Work out the finished part from the listing and answer in its coordinate system (mm). Round coordinates to 2 decimals unless told otherwise and drop trailing zeros. Order: outer loops, then holes, each group sorted by start corner. A loop starts at its lowest first (then second) coordinate and runs counter-clockwise, first axis right, second up. Notation, with made-up numbers: (-14.5, 15.5) -> (-10.5, 15.5) arc R21 ccw to (-10.5, 23.5) -> close; hole circle Ø6 at (8, -37). An arc over 180 degrees is marked (long way). Use one line per item in the form item = value.
```python
from build123d import *

# Parameters (mm, degrees)
F1_DEPTH = 1206.5


with BuildPart() as f1:
    # F0 (on Front) → F1 (new body)
    with BuildSketch(Plane.XZ):
        with BuildLine():
            Line((0, 38.1), (0, 0))
            Line((0, 0), (38.1, 0))
            ThreePointArc((38.1, 0), (37.170064, 2.245064), (34.925, 3.175))
            Line((34.925, 3.175), (3.175, 3.175))
            Line((3.175, 3.175), (3.175, 34.925))
            ThreePointArc((3.175, 34.925), (2.245064, 37.170064), (0, 38.1))
        make_face()
    extrude(amount=-F1_DEPTH)


solid = f1.part
```
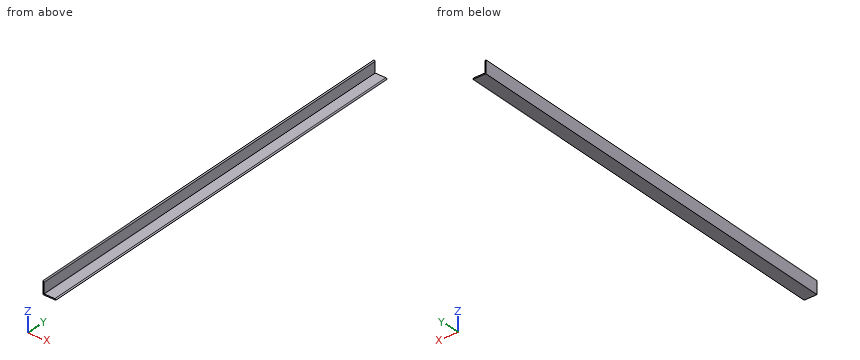
Item 1: Consider line 1 along X through (y, z) = (158, 19.5) (3 decimals). Determine where the line is inside the solid, lowest interval first.
Findings:
line_1 = 0 to 3.175
Item 2: Flat-ended cylindrical pins translate along their axes: P1, Ø12, axis at x = 16, z = 9.5, coming from the +Y side; P2, Ø2, axis at x = 25, y = 480, coming from the -Z side; P3, Ø16, axis at x = 13, y = 544.5, coming from the +Z side (3 decimals). Find the tip coordinate at first contact, or state that the pin passes through.
Findings:
P1 = through
P2 = 0
P3 = 3.175
Item 3: The part is cut by section A-A, the plane y = 553. Give the vertices of the cut face in (x, z) (3 decimals).
Findings:
outline = (0, 0) -> (38.1, 0) arc R3.175 ccw to (34.925, 3.175) -> (3.175, 3.175) -> (3.175, 34.925) arc R3.175 ccw to (0, 38.1) -> close
Item 4: The part is cut by section C-C, the plane z = 20. Give the vertices of the cut face in (x, y) (3 decimals).
Findings:
outline = (0, 0) -> (3.175, 0) -> (3.175, 1206.5) -> (0, 1206.5) -> close
Item 5: The part is cut by section B-B, the plane x = 11. Give the vertices of the cut face in (y, z) (3 decimals).
Findings:
outline = (0, 0) -> (1206.5, 0) -> (1206.5, 3.175) -> (0, 3.175) -> close
